```python
from build123d import *

# Parameters (mm, degrees)
BOSS_EXTRUDE1_DEPTH      = 11.1125
BOSS_EXTRUDE1_DEPTH_BACK = 11.1125
SKETCH3_R                = 6.6675
SKETCH3_R_2              = 4.7625
SKETCH4_R                = 4.7625
CUT_EXTRUDE1_DEPTH       = 27.587663165


with BuildPart() as part:
    # Sketch2 → Revolve1 (revolve)
    with BuildSketch(Plane(origin=(0, 0, 0), x_dir=(1, 0, 0), z_dir=(0, 1, 0))):
        with BuildLine():
            Line((0, 10.31875), (0, -10.31875))
            ThreePointArc((0, -10.31875), (10.31875, 0), (0, 10.31875))
        make_face()
    revolve(axis=Axis((0, 0, -10.31875), (0, 0, 1)))

    # Sketch3 → Boss-Extrude1 (add, two sides: drawn at the far end of the back side and taken through both)
    with BuildSketch(Plane(origin=(0, 0, 0), x_dir=(0, 0, -1), z_dir=(1, 0, 0)).offset(-BOSS_EXTRUDE1_DEPTH_BACK)):
        Circle(SKETCH3_R)
        Circle(SKETCH3_R_2, mode=Mode.SUBTRACT)
    extrude(amount=BOSS_EXTRUDE1_DEPTH + BOSS_EXTRUDE1_DEPTH_BACK)

    # Sketch4 → Cut-Extrude1 (cut, through all)
    with BuildSketch(Plane(origin=(11.1125, 0, 0), x_dir=(0, 0, -1), z_dir=(1, 0, 0))):
        Circle(SKETCH4_R)
    extrude(amount=-CUT_EXTRUDE1_DEPTH, mode=Mode.SUBTRACT)


solid = part.part
```
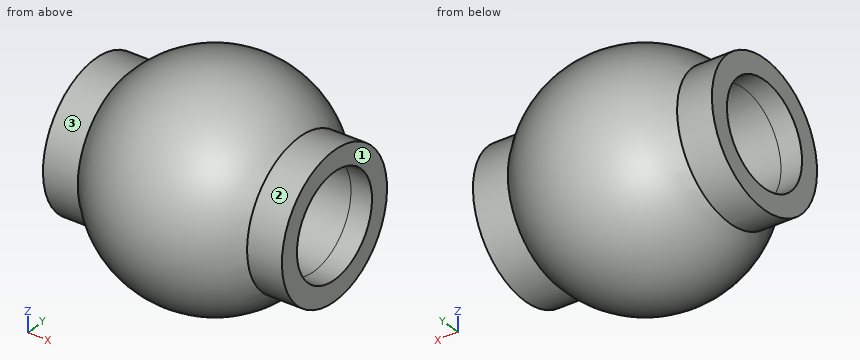
CAD build for the part. Positions are in the model's coordinates, mm. Face numbers are marked on the shaded views. A direction names the side the tool comes from. Coordinates: 2 decimals unless noted, no trailing zeros. Order: outer loops, then holes, each group sorted by start corner. A loop starts at its lowest first (then second) coordinate and runs counter-clockwise, first axis right, second up. Notation, with made-up numbers: M 34,58.5 L 49,58.5 A25 cw 49,72.5 Z; hole C -24.5,-40 d11. An arc over 180 degrees is marked long. Write each question's results on one line, items separated by ' | '. Start each with the question number.
Q1. Which spindle directions (+Z, -Z, +X, -X, +Y, -Y) get a long thin tool onto all of the face, cutting with end or side? Do the marked faces 1, 2 and 3. Say none if no direction does.
Q2. Cut at D-D (z = -5.75). List the corners of the cut face in (x, y), then the cut area to 3 significant figures.
Q3. Cut at A-A (y = 0). List the corners of the cut face in (x, z).
Q4. Drill centre lines: probe 1 along Y at (x, z) = (-10.2, 0); probe 2 along Y at (x, z) = (-3.75, 0). Where is each one in solid material? Low to high. Write a range as from..to.
Q5. Cut at C-C (x = -1). List the corners of the cut face in (y, z) (1 decimal).
Q6. Flat gauge pins, fed straight in: P1, Ø3, axis at x = -4, z = 3, coming from the +Y side; P2, Ø2, axis at x = -3.5, y = -1.5, coming from the +Z side; P3, Ø4, axis at x = -6, z = 7.5, coming from the -Y side. Where does each tip first touch, or does it go through?
Found:
1) face 1: +Z, -Z, +X, +Y, -Y | face 2: +X | face 3: -X
2) outline: M -11.11,-3.38 L -7.88,-3.38 A8.57 ccw 7.88,-3.38 L 11.11,-3.38 L 11.11,3.38 L 7.88,3.38 A8.57 ccw -7.88,3.38 L -11.11,3.38 Z | area: 268 mm²
3) outline: M -11.11,-6.67 L -7.88,-6.67 A10.32 ccw 7.88,-6.67 L 11.11,-6.67 L 11.11,-4.76 L -11.11,-4.76 Z; M -11.11,4.76 L 11.11,4.76 L 11.11,6.67 L 7.88,6.67 A10.32 ccw -7.88,6.67 L -11.11,6.67 Z
4) probe 1: -6.67..-4.76, 4.76..6.67 | probe 2: -9.61..-4.76, 4.76..9.61
5) outline: C 0,0 d20.5; hole C 0,0 d9.5
6) P1: y = 9.71 | P2: z = 9.93 | P3: y = -6.97
